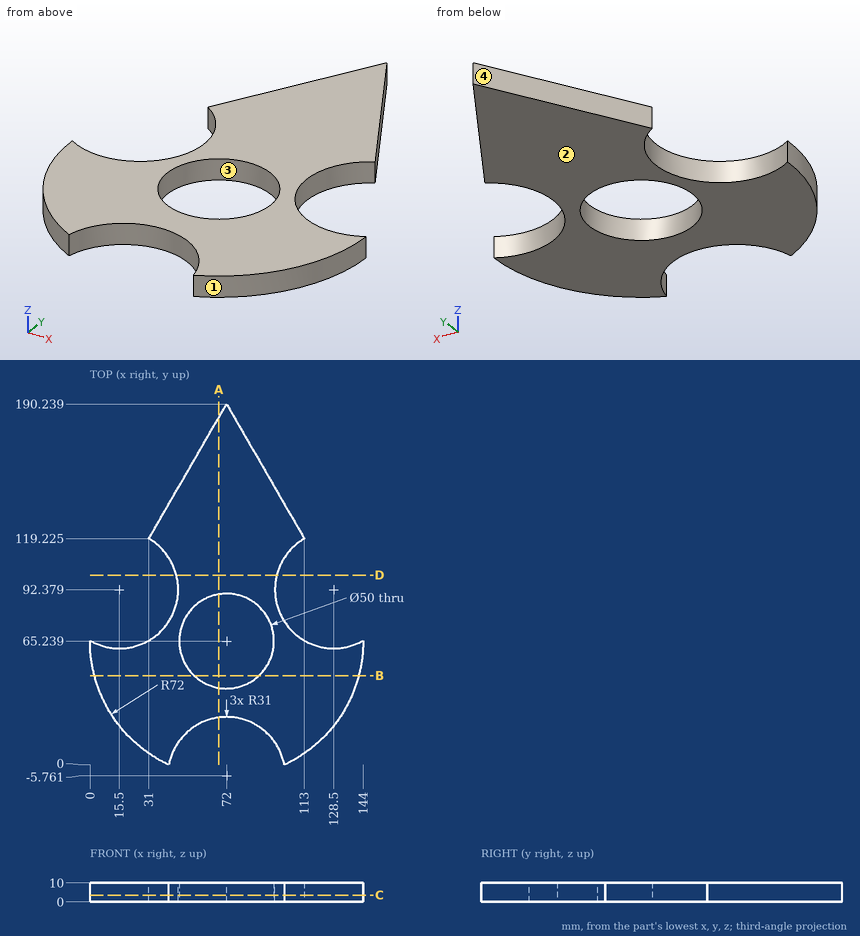
Print and shaded views of the part. All mm, measured from the part's lowest x, y and z. Give positions to 0.01 mm unless a question says otherwise; leave off trailing zeros. Write each loop counter-clockwise with the first axis right and the second up, starting at its lowest first coordinate (ties: lowest second). Pieces come first, ordered by that corner, then holes. Notation, with made-up numbers: (-7, 52) -> (11, 52) arc R31 ccw to (11, 85) -> close; hole circle Ø5 at (54.5, -31). An arc over 180 degrees is marked (long way). Write item = value, one per line.
(1) Slice it at C-C, the plane z = 3.5. Give the cut face in (x, y) (1 decimal).
Determined:
outline = (0, 65.5) arc R72 ccw to (41.5, 0) arc R31 cw to (102.5, 0) arc R72 ccw to (144, 65.5) arc R31 cw to (113, 119.2) -> (72, 190.2) -> (31, 119.2) arc R31 cw to start; hole circle Ø50 at (72, 65.2)
(2) Slice it at D-D, the plane y = 100. Give the cut face in (x, z), then the cut area to 3 significant figures.
Determined:
outline = (45.55, 0) -> (98.45, 0) -> (98.45, 10) -> (45.55, 10) -> close
area = 529 mm2
(3) Slice it at A-A, the plane x = 68. Give the cut face in (y, z).
Determined:
outline = (24.98, 0) -> (40.56, 0) -> (40.56, 10) -> (24.98, 10) -> close; (89.92, 0) -> (183.31, 0) -> (183.31, 10) -> (89.92, 10) -> close
(4) Probe line 1 along Y through (x, z) = (72, 3); line 2 along Y through (x, z) = (67, 4.25) (1 decimal); line 3 along X through (y, z) = (87, 8.25) (1 decimal). List the from-to ranges inside material, lowest first.
Determined:
line_1 = 25.24 to 40.24, 90.24 to 190.24
line_2 = 24.8 to 40.7, 89.7 to 181.6
line_3 = 46 to 59.7, 84.3 to 98
(5) Mould opens along X. For the marked faces 1, 2, 3 and 4 say: released by +X, released by -X, zero draft, split by the parting line, or undercut.
Determined:
face_1 = released by +X
face_2 = zero draft
face_3 = undercut
face_4 = released by -X
(6) Slice it at B-B, the plane y = 47. Give the cut face in (x, z).
Determined:
outline = (2.35, 0) -> (54.9, 0) -> (54.9, 10) -> (2.35, 10) -> close; (89.1, 0) -> (141.65, 0) -> (141.65, 10) -> (89.1, 10) -> close
(7) Flat gauge pins, fed straight in: P1, Ø5, axis at x = 35.5, z = 2, coming from the -Y side; P2, Ø2, axis at x = 126.5, z = 5.5, coming from the +Y side; P3, Ø2, axis at y = 139.5, z = 5, coming from the +X side. Where does each tip first touch, or does it go through?
Determined:
P1 = 1.77
P2 = 61.52
P3 = 101.87
